Work out the finished part from the listing and answer in its coordinate system (mm). Face numbers are marked on the shaded views. A direction names the side the tool comes from. Round coordinates to 2 decimals unless told otherwise and drop trailing zeros. Order: outer loops, then holes, each group sorted by start corner. A loop starts at its lowest first (then second) coordinate and runs counter-clockwise, first axis right, second up. Notation, with made-up numbers: M -36,55 L 16,55 A26 ccw 16,82 Z; hole C 61.25,-14 d7. An arc over 180 degrees is marked long. Return JSON: item names as keys, results as strings.
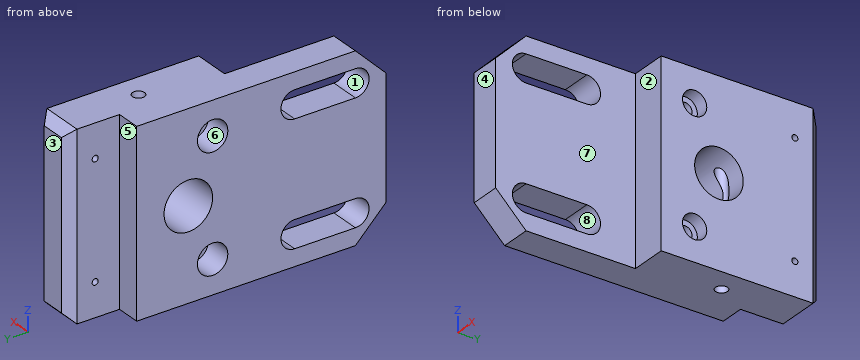
from build123d import *

# Parameters (mm, degrees)
EXTRUDE_1_DEPTH              = 30
CUT_EXTRUDE_1_DEPTH          = 23
HOLE_WIZARD_M4_1_D           = 4.5
HOLE_WIZARD_M4_1_CBORE_D     = 8
HOLE_WIZARD_M4_1_CBORE_DEPTH = 4.4
SKETCH_6_R                   = 5
CUT_EXTRUDE_2_DEPTH          = 9
SKETCH_7_R                   = 8
CUT_EXTRUDE_3_DEPTH          = 23
HOLE_WIZARD_M4_1_2_D         = 2
HOLE_WIZARD_M4_2_D           = 4
CHAMFER_1_SIZE               = 10
CHAMFER_2_SIZE               = 3


with BuildPart() as part:
    # 스케치1 → 보스-돌출1 (new body, symmetric)
    with BuildSketch(Plane.XY):
        Polygon((0, 0), (0, 82), (8, 82), (8, 99), (22, 99), (22, 46), (10, 46), (10, 0), align=None)
    extrude(amount=EXTRUDE_1_DEPTH, both=True)

    # 스케치2 → 컷-돌출1 (cut, through all)
    with BuildSketch(Plane.ZY):
        with BuildLine():
            Line((-15.5, 30), (-15.5, 10))
            ThreePointArc((-15.5, 10), (-20, 5.5), (-24.5, 10))
            Line((-24.5, 10), (-24.5, 30))
            ThreePointArc((-24.5, 30), (-20, 34.5), (-15.5, 30))
        make_face()
        with BuildLine():
            Line((15.5, 30), (15.5, 10))
            ThreePointArc((15.5, 10), (20, 5.5), (24.5, 10))
            Line((24.5, 10), (24.5, 30))
            ThreePointArc((24.5, 30), (20, 34.5), (15.5, 30))
        make_face()
    extrude(amount=-CUT_EXTRUDE_1_DEPTH, mode=Mode.SUBTRACT)

    # Hole Wizard M4 _ _ _ _ _1 (through all)
    with Locations(Plane(origin=(22, 0, 0), x_dir=(0, 0, -1), z_dir=(1, 0, 0))):
        with Locations((-19, 57), (19, 57)):
            CounterBoreHole(HOLE_WIZARD_M4_1_D / 2, HOLE_WIZARD_M4_1_CBORE_D / 2, HOLE_WIZARD_M4_1_CBORE_DEPTH)

    # 스케치6 → 컷-돌출2 (cut)
    with BuildSketch(Plane.ZY):
        with Locations((-19, 57)):
            Circle(SKETCH_6_R)
        with Locations((19, 57)):
            Circle(SKETCH_6_R)
    extrude(amount=-CUT_EXTRUDE_2_DEPTH, mode=Mode.SUBTRACT)

    # 스케치7 → 컷-돌출3 (cut, through all)
    with BuildSketch(Plane(origin=(22, 0, 0), x_dir=(0, 0, -1), z_dir=(1, 0, 0))):
        with Locations((0, 65)):
            Circle(SKETCH_7_R)
    extrude(amount=-CUT_EXTRUDE_3_DEPTH, mode=Mode.SUBTRACT)

    # Hole Wizard M4 _ _1 2 (through all)
    with Locations(Plane(origin=(22, 0, 0), x_dir=(0, 0, -1), z_dir=(1, 0, 0))):
        with Locations((-19, 90), (19, 90)):
            Hole(HOLE_WIZARD_M4_1_2_D / 2)

    # M4 여유 구멍2 (through all)
    with Locations(Plane.XY.offset(30)):
        with Locations((14, 71.5)):
            Hole(HOLE_WIZARD_M4_2_D / 2)

    # 모따기1
    chamfer_1_edges = [part.edges().sort_by_distance(p)[0] for p in [
        (5, 0, -30),
        (5, 0, 30),
    ]]
    chamfer(chamfer_1_edges, length=CHAMFER_1_SIZE)

    # 모따기2
    chamfer_2_edges = [part.edges().sort_by_distance(p)[0] for p in [
        (8, 99, 0),
        (22, 99, 0),
        (15, 99, 30),
        (15, 99, -30),
    ]]
    chamfer(chamfer_2_edges, length=CHAMFER_2_SIZE)


solid = part.part
Item 1: Which of the six approach directions +Z, -Z, +X, -X, +Y, -Y give full straight-line access (tool end or side, diameter ignored) to the marked faces 4, 5, 6, 7 and 8?
Output:
{"face 4": "+Z, -Z, +X, -X, -Y", "face 5": "+Z, -Z, -X, +Y", "face 6": "-X", "face 7": "+Z, -Z, +X, -Y", "face 8": "+X, -X"}
Item 2: Find section D-D (z = -19). State how many separate pieces and enclosed holes the cut face has, plus the area to 3 significant figures.
Output:
{"separate pieces": "4", "enclosed holes": "1", "area": "989 mm^2"}
Item 3: Find section C-C (x = 14). Determine the outline of the cut face in (y, z), plus the area to 3 significant figures.
Output:
{"outline": "M 46,-30 L 69.5,-30 L 69.5,-6.61 A8 cw long 69.5,6.61 L 69.5,30 L 46,30 Z; M 73.5,-30 L 96,-30 L 99,-27 L 99,27 L 96,30 L 73.5,30 Z; hole C 57,-19 d4.5; hole C 57,19 d4.5; hole C 90,-19 d2; hole C 90,19 d2", "area": "2,720 mm^2"}
Item 4: The mould has two halves that part along Y. Classify the marked faces 1, 2 and 3: pulls with the +Y half, pulls with the -Y half, needs draft (parallel to the pull), parting line crosses it, or undercut.
Output:
{"face 1": "undercut", "face 2": "pulls with the -Y half", "face 3": "pulls with the +Y half"}
Item 5: Find section B-B (z = 7). Determine the outline of the cut face in (x, y), plus the area to 3 significant figures.
Output:
{"outline": "M 0,0 L 10,0 L 10,46 L 22,46 L 22,61.13 L 0,61.13 Z; M 0,68.87 L 22,68.87 L 22,96 L 19,99 L 11,99 L 8,96 L 8,82 L 0,82 Z; hole C 14,71.5 d4", "area": "1,300 mm^2"}
Item 6: Consider line 1 along Y through (x, z) = (18.5, -19); line 2 along Z through (x, y) = (4.5, 10.5); line 3 along Z through (x, y) = (15.75, 90). Determine where each line is inside the solid, lowest interval first. Write a range as [from, to].
Output:
{"line 1": "y = [46, 53], [61, 89], [91, 99]", "line 2": "z = [-30, -24.5], [-15.5, 15.5], [24.5, 30]", "line 3": "z = [-30, -20], [-18, 18], [20, 30]"}
Item 7: Each of these flat-tipped pins is pushed along its axis until it touches: pin 1 (4 mm diameter, centred on x = 15, z = 21.5, fed in from -Y); pin 2 (5 mm diameter, centred on y = 56.5, z = 17, fed in from -X); pin 3 (4 mm diameter, centred on y = 56, z = 20.5, fed in from +X). Where does it stop, or does it pass through?
Output:
{"pin 1": "stops at y = 46", "pin 2": "stops at x = 9", "pin 3": "stops at x = 17.6"}
Item 8: Find section A-A (y = 65). Determine the outline of the cut face in (x, z), plus the area to 3 significant figures.
Output:
{"outline": "M 0,-30 L 22,-30 L 22,-8 L 0,-8 Z; M 0,8 L 22,8 L 22,30 L 0,30 Z", "area": "968 mm^2"}
